```python
from build123d import *

# Parameters (mm, degrees)
BOSS_EXTRUDE1_DEPTH   = 75
CHAMFER1_SIZE         = 0.5
CHAMFER1_SIZE2        = 0.288675135
CHAMFER1_PART_2_SIZE  = 0.5
CHAMFER1_PART_2_SIZE2 = 0.288675135
CHAMFER1_PART_3_SIZE  = 0.5
CHAMFER1_PART_3_SIZE2 = 0.288675135
CHAMFER1_PART_4_SIZE  = 0.5
CHAMFER1_PART_4_SIZE2 = 0.288675135
SKETCH2_R             = 1.75
CUT_EXTRUDE1_DEPTH    = 8
SKETCH3_R             = 3
CUT_EXTRUDE2_DEPTH    = 4.5
LPATTERN1_COUNT       = 6
LPATTERN1_PITCH       = 25


with BuildPart() as part:
    # Sketch1 → Boss-Extrude1 (new body, symmetric)
    with BuildSketch(Plane.XY):
        with BuildLine():
            Line((-6, -4), (6, -4))
            Line((6, -4), (6, 0.3))
            ThreePointArc((6, 0.3), (4.8, 1.5), (6, 2.7))
            Line((6, 2.7), (6, 4))
            Line((6, 4), (-6, 4))
            Line((-6, 4), (-6, 2.7))
            ThreePointArc((-6, 2.7), (-4.8, 1.5), (-6, 0.3))
            Line((-6, 0.3), (-6, -4))
        make_face()
    extrude(amount=BOSS_EXTRUDE1_DEPTH, both=True)

    # Chamfer1
    chamfer1_edges = [part.edges().sort_by_distance(p)[0] for p in [
        (6, -4, 0),
    ]]
    chamfer1_side = [part.faces().sort_by_distance(p)[0] for p in [
        (0, -4, 0),
    ]]
    chamfer(chamfer1_edges, length=CHAMFER1_SIZE, length2=CHAMFER1_SIZE2, reference=chamfer1_side[0])

    # Chamfer1 part 2
    chamfer1_part_2_edges = [part.edges().sort_by_distance(p)[0] for p in [
        (-6, -4, 0),
    ]]
    chamfer1_part_2_side = [part.faces().sort_by_distance(p)[0] for p in [
        (-6, -1.85, 0),
    ]]
    chamfer(chamfer1_part_2_edges, length=CHAMFER1_PART_2_SIZE, length2=CHAMFER1_PART_2_SIZE2, reference=chamfer1_part_2_side[0])

    # Chamfer1 part 3
    chamfer1_part_3_edges = [part.edges().sort_by_distance(p)[0] for p in [
        (-6, 4, 0),
    ]]
    chamfer1_part_3_side = [part.faces().sort_by_distance(p)[0] for p in [
        (0, 4, 0),
    ]]
    chamfer(chamfer1_part_3_edges, length=CHAMFER1_PART_3_SIZE, length2=CHAMFER1_PART_3_SIZE2, reference=chamfer1_part_3_side[0])

    # Chamfer1 part 4
    chamfer1_part_4_edges = [part.edges().sort_by_distance(p)[0] for p in [
        (6, 4, 0),
    ]]
    chamfer1_part_4_side = [part.faces().sort_by_distance(p)[0] for p in [
        (6, 3.35, 0),
    ]]
    chamfer(chamfer1_part_4_edges, length=CHAMFER1_PART_4_SIZE, length2=CHAMFER1_PART_4_SIZE2, reference=chamfer1_part_4_side[0])

    # Sketch2 → Cut-Extrude1 (cut)
    with BuildSketch(Plane(origin=(0, 4, 0), x_dir=(1, 0, 0), z_dir=(0, 1, 0))):
        with Locations((0.088052027, -62.5)):
            Circle(SKETCH2_R)
    cut_extrude1 = extrude(amount=-CUT_EXTRUDE1_DEPTH, mode=Mode.SUBTRACT)

    # Sketch3 → Cut-Extrude2 (cut)
    with BuildSketch(Plane(origin=(0, 4, 0), x_dir=(1, 0, 0), z_dir=(0, 1, 0))):
        with Locations((0.088052027, -62.5)):
            Circle(SKETCH3_R)
    cut_extrude2 = extrude(amount=-CUT_EXTRUDE2_DEPTH, mode=Mode.SUBTRACT)

    # LPattern1: Cut-Extrude1, Cut-Extrude2 ×6
    with Locations(*[(0, 0, -i * LPATTERN1_PITCH) for i in range(1, LPATTERN1_COUNT)]):
        add(cut_extrude1, mode=Mode.SUBTRACT)
        add(cut_extrude2, mode=Mode.SUBTRACT)


solid = part.part
```
Work out the finished part from the listing and answer in its coordinate system (mm). A direction names the side the tool comes from. Give positions to 0.01 mm unless a question says otherwise; leave off trailing zeros. Loops run counter-clockwise (first coordinate to the right, second up) from the corner with the lowest first, then second, coordinate; pieces in that order, holes last. Notation, with made-up numbers: (40, 79.5) -> (62, 79.5) arc R17 cw to (62, 99.5) -> close; hole circle Ø6 at (-6.5, 79). An arc over 180 degrees is marked (long way). Write item = value, one per line. Start each with the question number.
(1) Which of the six approach directions +Z, -Z, +X, -X, +Y, -Y give full straight-line access (tool end or side, diameter ignored) to faces 4 (the flat face through (0, -4, 1)), 5 (the cylindrical face through (-0.302, 1.781, -40.474))?
(2) Given pin 1 Ø5.5 at (x, z) = (0.09, 37.5) entering from +Y; pin 2 Ø2 at (x, z) = (0.09, 37.5) entering from +Y, each flat-ended and moving along its own axis, determine where each tip first touches the part or whether it passes through.
(3) Find the intervals of material crossed by probe 1 along Y at (x, z) = (0.75, -60.5); probe 2 along X at (y, z) = (-1, 63.5); probe 3 along X at (y, z) = (1.25, -63.5), in increasing order. Write a range as from..to.
(4) Find section C-C on z = 31.5. Give the vertices of the cut face in (x, y).
(5) Find section B-B on y = -2.25. Give the vertices of the cut face in (x, z), and give its area (3 significant figures).
(6) Find section A-A on z = 12.5. Give the vertices of the cut face in (x, y), and give its area (3 significant figures).
(7) The mould has two halves that part along X. Classify faces 1 (the flat face through (-6, -2, 1)), 2 (the cylindrical face through (-2.12, 1.78, 10.47)), 3 (the flat face through (6, -2, 1)): +X half, -X half, draft (parallel to the pull), parting line (faces both ways), or undercut.
From the geometry:
q1.face_4 = +Z, -Z, +X, -X, -Y
q1.face_5 = +Y
q2.pin_1 = -0.5
q2.pin_2 = through
q3.probe_1 = -4..-0.5
q3.probe_2 = -6..-1.35, 1.52..6
q3.probe_3 = -4.83..-2.74, 2.92..4.83
q4.outline = (-6, -3.5) -> (-5.71, -4) -> (5.5, -4) -> (6, -3.71) -> (6, 0.3) arc R1.2 cw to (6, 2.7) -> (6, 3.5) -> (5.71, 4) -> (-5.5, 4) -> (-6, 3.71) -> (-6, 2.7) arc R1.2 cw to (-6, 0.3) -> close
q5.outline = (-6, -75) -> (6, -75) -> (6, 75) -> (-6, 75) -> close; hole circle Ø3.5 at (0.09, -62.5); hole circle Ø3.5 at (0.09, -37.5); hole circle Ø3.5 at (0.09, -12.5); hole circle Ø3.5 at (0.09, 12.5); hole circle Ø3.5 at (0.09, 37.5); hole circle Ø3.5 at (0.09, 62.5)
q5.area = 1,740 mm^2
q6.outline = (-6, -3.5) -> (-5.71, -4) -> (-1.66, -4) -> (-1.66, -0.5) -> (-2.91, -0.5) -> (-2.91, 4) -> (-5.5, 4) -> (-6, 3.71) -> (-6, 2.7) arc R1.2 cw to (-6, 0.3) -> close; (1.84, -4) -> (5.5, -4) -> (6, -3.71) -> (6, 0.3) arc R1.2 cw to (6, 2.7) -> (6, 3.5) -> (5.71, 4) -> (3.09, 4) -> (3.09, -0.5) -> (1.84, -0.5) -> close
q6.area = 51.9 mm^2
q7.face_1 = -X half
q7.face_2 = undercut
q7.face_3 = +X half
